```python
from build123d import *


with BuildPart() as f1:
    # F0 (on Front) → F1 (revolve)
    with BuildSketch(Plane.XZ):
        with BuildLine():
            Line((0, 141), (0, 0))
            Line((0, 0), (16, 0))
            Line((16, 0), (16, 115))
            Line((16, 115), (50, 115))
            Line((50, 115), (50, 120))
            Line((50, 120), (16, 120))
            ThreePointArc((16, 120), (19.252662, 129.327381), (27.600006, 134.609587))
            Line((27.600006, 134.609587), (27.600006, 150))
            Line((27.600006, 150), (8, 150))
            Line((8, 150), (8, 141))
            Line((8, 141), (0, 141))
        make_face()
    revolve(axis=Axis((0, 0, 70.5), (0, 0, 1)))


solid = f1.part
```
Geometry check sheet. Reference: the model listing, model coordinates, mm. A direction names the side the tool comes from. Give positions to 0.01 mm unless a question says otherwise; leave off trailing zeros. Write each loop counter-clockwise with the first axis right and the second up, starting at its lowest first coordinate (ties: lowest second). Pieces come first, ordered by that corner, then holes. Notation, with made-up numbers: (28.25, 36) -> (40.25, 36) arc R11 cw to (40.25, 40) -> close; hole circle Ø2 at (30.25, -16.5). An arc over 180 degrees is marked (long way). One line per question, with ' | ' between items.
Item 1: Scan lines: line 1 along Y through (x, z) = (0, 144); line 2 along Z through (x, y) = (-42.5, -10.5); line 3 along Z through (x, y) = (20.5, 5). Record each from-to range of solid material in increasing order.
Determined:
line 1: -27.6 to -8, 8 to 27.6 | line 2: 115 to 120 | line 3: 115 to 120, 131.27 to 150
Item 2: Depth check by flat-ended pin: pin 1 (8 mm diameter, centred on y = 6, z = 105.5, fed in from +X); pin 2 (5 mm diameter, centred on x = 2.5, y = 2, fed in from +Z); pin 3 (12 mm diameter, centred on x = -35.5, z = 123, fed in from +Y). Enter the tip coordinate at first touch or a pass-through.
Determined:
pin 1: x = 15.87 | pin 2: z = 141 | pin 3: y = 39.77
Item 3: Sectioned sample at D-D, the plane z = 106. Record the boundary of the cut face in (x, y), plus the area to 3 significant figures.
Determined:
outline: circle Ø32 at (0, 0) | area: 804 mm^2
Item 4: Sectioned sample at A-A, the plane x = 0. Record the boundary of the cut face in (y, z).
Determined:
outline: (-50, 115) -> (-16, 115) -> (-16, 0) -> (16, 0) -> (16, 115) -> (50, 115) -> (50, 120) -> (16, 120) arc R15 cw to (27.6, 134.61) -> (27.6, 150) -> (8, 150) -> (8, 141) -> (-8, 141) -> (-8, 150) -> (-27.6, 150) -> (-27.6, 134.61) arc R15 cw to (-16, 120) -> (-50, 120) -> close
Item 5: Draft check along X on faces 1 (the flat face through (12, 12, 115)), 2 (the cylindrical face through (-1.73, -7.81, 145.44)), 3 (the cylindrical face through (-3.593, 27.365, 142.413)), 4 (the flat face through (0, 0, 141)). Enter one of: released by +X, released by -X, zero draft, split by the parting line, or undercut.
Determined:
face 1: zero draft | face 2: undercut | face 3: split by the parting line | face 4: undercut
Item 6: Access from +Z, -Z, +X, -X, +Y, -Y to the whole of each face (thin tool, end or side, straight path). Record for faces 5 (the cylindrical face through (-3.47, -15.62, 58.3)), 6 (the cylindrical face through (47.69, 15.02, 117.54)), 7 (the flat face through (-12, 12, 120)).
Determined:
face 5: -Z | face 6: +Z, -Z | face 7: none
Item 7: Sectioned sample at C-C, the plane z = 139. Record the boundary of the cut face in (x, y), plus the area to 3 significant figures.
Determined:
outline: circle Ø55.2 at (0, 0) | area: 2,390 mm^2
